Drawing for the job (mm, zero at the part's lowest x, y, z). A direction names the side the tool comes from. Coordinates: 2 decimals unless noted, no trailing zeros. Write each loop counter-clockwise with the first axis right and the second up, starting at its lowest first coordinate (ties: lowest second). Pieces come first, ordered by that corner, then holes. Notation, with made-up numbers: M 9.25,-2 L 23.25,-2 A9 ccw 23.25,7 Z; hole C -8,-5.5 d2. An arc over 180 degrees is marked long. Put each result on its own line as item: value. Start each with the question number.
Q1. Cut at C-C (y = 2.1). Write the cut outline in (x, z), then the cut area to 3 significant figures.
Q2. Pull direction Y, two halves, no side cores. Call the marked faces 1, 2 and 3: pulls with the +Y half, pulls with the -Y half, needs draft (parallel to the pull), parting line crosses it, or undercut.
Q3. Which spindle directions (+Z, -Z, +X, -X, +Y, -Y) get a long thin tool onto all of the face, cutting with end or side? Do the marked faces 4, 5 and 6. Say none if no direction does.
Q4. Cut at B-B (x = 4.5). Write the cut outline in (y, z).
Q5. Cut at D-D (x = 2.75). Write the cut outline in (y, z), then the cut area to 3 significant figures.
Q6. Cut at A-A (z = 4.5). Write the cut outline in (x, y).
Q7. Drop flat-ended pins along their axis: pin 1 (1 mm diameter, centred on y = 2, z = 3.5, fed in from -X); pin 2 (2 mm diameter, centred on y = 2.5, z = 5.5, fed in from -X). Give the stop position or say it passes through.
Q8. Drill centre lines: line 1 along Z through (x, y) = (4.5, 1.35); line 2 along Y through (x, z) = (1.25, 6); line 3 along Z through (x, y) = (3.5, 3.5). Where is each one in solid material? Low to high.
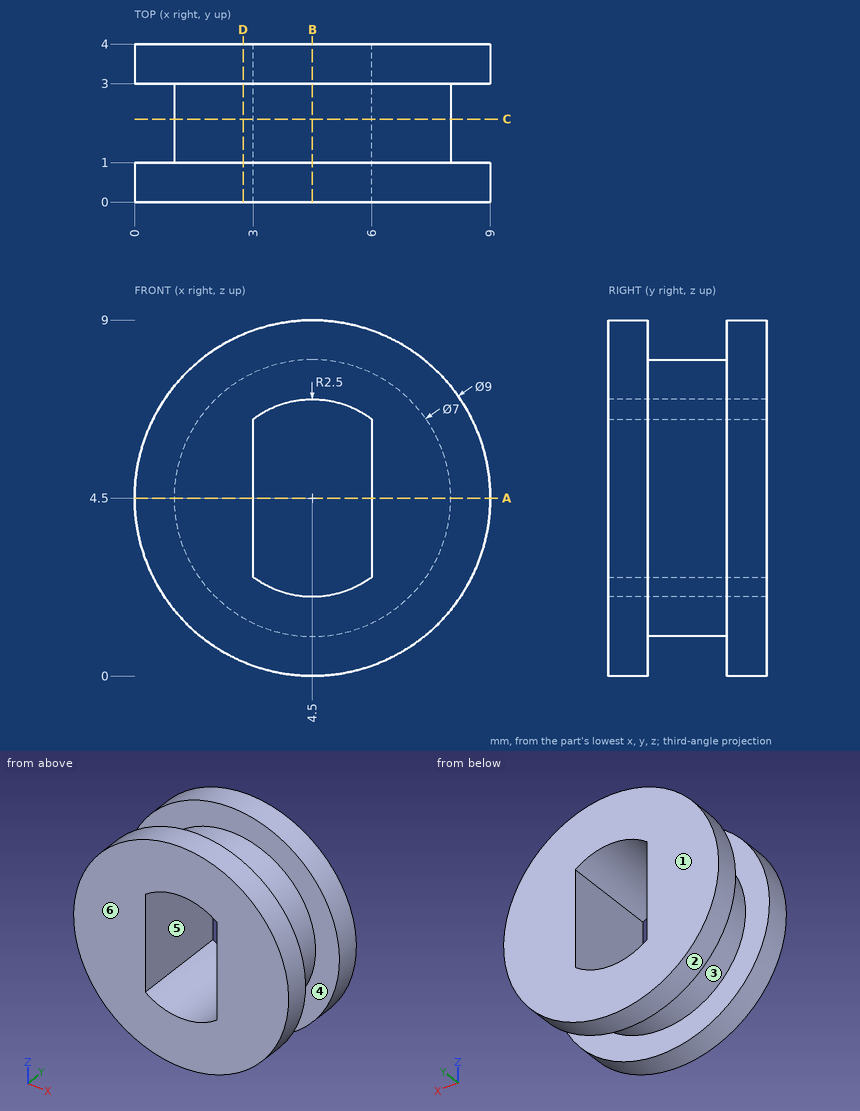
Computed values:
1. outline: C 4.5,4.5 d7; hole M 3,2.5 A2.5 ccw 6,2.5 L 6,6.5 A2.5 ccw 3,6.5 Z
1. area: 24.4 mm2
2. face 1: pulls with the +Y half
2. face 2: needs draft
2. face 3: undercut
3. face 4: none
3. face 5: +Y, -Y
3. face 6: +Z, -Z, +X, -X, -Y
4. outline: M 0,0 L 1,0 L 1,1 L 3,1 L 3,0 L 4,0 L 4,2 L 0,2 Z; M 0,7 L 4,7 L 4,9 L 3,9 L 3,8 L 1,8 L 1,9 L 0,9 Z
5. outline: M 0,0.35 L 1,0.35 L 1,1.47 L 3,1.47 L 3,0.35 L 4,0.35 L 4,8.65 L 3,8.65 L 3,7.53 L 1,7.53 L 1,8.65 L 0,8.65 Z
5. area: 28.7 mm2
6. outline: M 0,0 L 3,0 L 3,4 L 0,4 L 0,3 L 1,3 L 1,1 L 0,1 Z; M 6,0 L 9,0 L 9,1 L 8,1 L 8,3 L 9,3 L 9,4 L 6,4 Z
7. pin 1: x = 1.04
7. pin 2: x = 0
8. line 1: 1 to 2, 7 to 8
8. line 2: 0 to 1, 3 to 4
8. line 3: 0.11 to 2.21, 6.79 to 8.89
